For this review, use the dimensioned drawing (mm, ordinates from the lowest corner) and the shaded views. Coordinates: 2 decimals unless noted, no trailing zeros. Answer as CSV lines item,"result". Start each with the question number.
Q1. Wall thickness on L1, parallel to Z at x = 9, y = 13; L2, parallel to X at y = 24, z = 13; L3, parallel to Y at x = 21.5, z = 33: over which ranges is each line inside the solid? List them lowest first. Write a range as [from, to].
Q2. Consider section A-A on y = 22.75. State how many separate pieces and enclosed holes the cut face has, and give its area (4 significant figures).
Q3. For P1, Ø4, axis at x = 35.72, z = 22.22, coming from the +Y side, flat-tipped, find the tip position at first contact; note if it passes through.
Q4. The part is to be moulded in two halves that separate along X. For the marked faces 1, 2 and 3, say which applies: +X half, -X half, draft (parallel to the pull), parting line (faces both ways), or undercut.
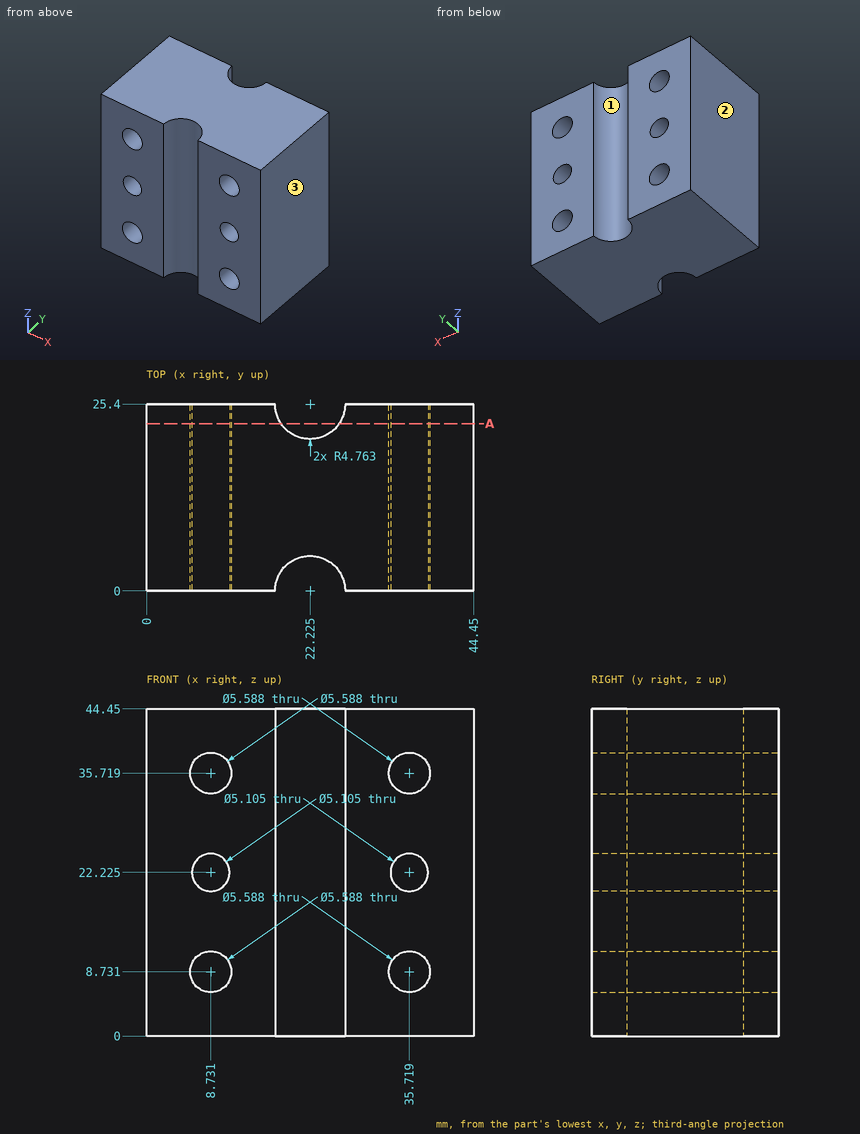
Evaluation:
1,L1,"z = [0, 5.95], [11.51, 19.69], [24.76, 32.94], [38.5, 44.45]"
1,L2,"x = [0, 17.67], [26.78, 44.45]"
1,L3,"y = [4.71, 20.69]"
2,separate pieces,"2"
2,enclosed holes,"6"
2,area,"1,485 mm²"
3,P1,"passes through"
4,face 1,"undercut"
4,face 2,"-X half"
4,face 3,"+X half"
